```python
from build123d import *

# Parameters (mm, degrees)
F1_W      = 100
F1_H      = 50
F2_DEPTH  = 15
F3_W      = 40
F3_H      = 5
F4_DEPTH  = 50
F5_T      = -3
F6_W      = 44
F6_H      = 12
F7_DEPTH  = 3
F9_W      = 10
F9_H      = 10
F10_DEPTH = 15.001
F11_R     = 5


with BuildPart() as f2:
    # F1 (on Top) → F2 (new body)
    with BuildSketch(Plane.XY):
        with Locations((50, 25)):
            Rectangle(F1_W, F1_H)
    extrude(amount=F2_DEPTH)

    # F3 (on Front) → F4 (cut, through all)
    with BuildSketch(Plane.XZ):
        with Locations((50, 12.5)):
            Rectangle(F3_W, F3_H)
    extrude(amount=-F4_DEPTH, mode=Mode.SUBTRACT)

    # F5
    f5_openings = [f2.faces().sort_by_distance(p)[0] for p in [
        (50, 25, 0),
    ]]
    offset(amount=F5_T, openings=f5_openings, kind=Kind.INTERSECTION)

    # F6 (on face) → F7 (cut, through all)
    with BuildSketch(Plane(origin=(0, 0, 0), x_dir=(0, -1, 0), z_dir=(-1, 0, 0))):
        with Locations((-25, 6)):
            Rectangle(F6_W, F6_H)
    extrude(amount=-F7_DEPTH, mode=Mode.SUBTRACT)

    # F9 (on offset) → F10 (cut, through all)
    with BuildSketch(Plane.XY.offset(15)):
        with Locations((80, 40)):
            Rectangle(F9_W, F9_H)
        with Locations((80, 10)):
            Rectangle(F9_W, F9_H)
        with Locations((80.0488266349, 25)):
            Rectangle(F9_W, F9_H)
        with Locations((20, 40)):
            Rectangle(F9_W, F9_H)
        with Locations((19.9511733651, 25)):
            Rectangle(F9_W, F9_H)
        with Locations((20, 10)):
            Rectangle(F9_W, F9_H)
        with Locations((60, 40)):
            Rectangle(F9_W, F9_H)
        with Locations((60, 10)):
            Rectangle(F9_W, F9_H)
        with Locations((40, 40)):
            Rectangle(F9_W, F9_H)
        with Locations((40, 10)):
            Rectangle(F9_W, F9_H)
    extrude(amount=-F10_DEPTH, mode=Mode.SUBTRACT)

    # F11
    f11_edges = [f2.edges().sort_by_distance(p)[0] for p in [
        (100, 0, 7.5),
        (100, 50, 7.5),
    ]]
    fillet(f11_edges, radius=F11_R)


solid = f2.part
```
Design review of the part built by this model. Coordinates are the model's own, in mm. A direction names the side the tool comes from. Coordinates: 2 decimals unless noted, no trailing zeros. Order: outer loops, then holes, each group sorted by start corner. A loop starts at its lowest first (then second) coordinate and runs counter-clockwise, first axis right, second up.
1) For faces 1 (the flat face through (20, 30, 14)), 2 (the flat face through (30, 25, 12)), list the 3-axis set-ups (+Z, -Z, +X, -X, +Y, -Y) from which the entire face can be reached by the end or side of a thin tool; tool diameter is ignored.
2) Mouldability with a two-part tool opening along X and no side actions: class faces 3 (the flat face through (50, 25, 7)), 4 (the flat face through (20, 35, 14)) as +X half, -X half, draft (parallel to the pull), parting line (faces both ways), or undercut.
3) Take a section at D-D, the plane y = 28.5. Give the boundary of the cut face in (x, z).
4) Take a section at A-A, the plane z = 13. State how many separate pieces and enclosed holes the cut face has, and give its area (3 significant figures).
5) Clearance check with flat-ended pins moving along their axes: pin 1 (1.5 mm diameter, centred on x = 86.5, y = 16, fed in from -Z); pin 2 (12 mm diameter, centred on x = 46.5, y = 30.5, fed in from +Z); pin 3 (5 mm diameter, centred on x = 31.5, y = 22, fed in from -Z). State where each tip first meets the part, or that it passes through.
6) Take a section at B-B, the plane x = 22. Give the boundary of the cut face in (y, z), and give its area (3 significant figures).
7) Wall thickness on line 1 along X through (y, z) = (10, 11.5); line 2 along X through (y, z) = (6, 12.5); line 3 along X through (y, z) = (43, 7.25): over which ranges is each line inside the solid? List them lowest first.
Returned:
1. face 1: +Z, -Z
1. face 2: +Z, +Y, -Y
2. face 3: draft
2. face 4: undercut
3. outline: (0, 12) - (14.95, 12) - (14.95, 15) - (0, 15) - close; (24.95, 12) - (27, 12) - (27, 7) - (73, 7) - (73, 12) - (75.05, 12) - (75.05, 15) - (70, 15) - (70, 10) - (30, 10) - (30, 15) - (24.95, 15) - close; (85.05, 12) - (97, 12) - (97, 0) - (100, 0) - (100, 15) - (85.05, 15) - close
4. separate pieces: 2
4. enclosed holes: 6
4. area: 2,390 mm2
5. pin 1: stops at z = 12
5. pin 2: stops at z = 10
5. pin 3: stops at z = 7
6. outline: (0, 0) - (3, 0) - (3, 12) - (5, 12) - (5, 15) - (0, 15) - close; (15, 12) - (20, 12) - (20, 15) - (15, 15) - close; (30, 12) - (35, 12) - (35, 15) - (30, 15) - close; (45, 12) - (47, 12) - (47, 0) - (50, 0) - (50, 15) - (45, 15) - close
6. area: 132 mm2
7. line 1: x = 27 to 30, 70 to 73, 97 to 100
7. line 2: x = 0 to 15, 25 to 30, 70 to 75, 85 to 100
7. line 3: x = 27 to 35, 45 to 55, 65 to 73, 97 to 100
